from build123d import *

# Parameters (mm, degrees)
SKETCH008_W     = 217
SKETCH008_H     = 40
SKETCH008_W_2   = 214.6
SKETCH008_H_2   = 37.6
PAD006_DEPTH    = 50
SKETCH009_W     = 224.6
SKETCH009_H     = 47.6
SKETCH009_W_2   = 214.6
SKETCH009_H_2   = 37.6
PAD007_DEPTH    = 30
SKETCH010_W     = 224.6
SKETCH010_H     = 20
PAD008_DEPTH    = 5
POCKET001_DEPTH = 87.601
PAD009_DEPTH    = 3
PAD010_DEPTH    = 3


with BuildPart() as part:
    # Sketch008 → Pad006 (new body)
    with BuildSketch(Plane.XY):
        Rectangle(SKETCH008_W, SKETCH008_H)
        Rectangle(SKETCH008_W_2, SKETCH008_H_2, mode=Mode.SUBTRACT)
    extrude(amount=PAD006_DEPTH)

    # Sketch009 → Pad007 (join)
    with BuildSketch(Plane.XY):
        Rectangle(SKETCH009_W, SKETCH009_H)
        Rectangle(SKETCH009_W_2, SKETCH009_H_2, mode=Mode.SUBTRACT)
    extrude(amount=PAD007_DEPTH)

    # Sketch010 → Pad008 (join)
    with BuildSketch(Plane.XY):
        with Locations((0, 33.8)):
            Rectangle(SKETCH010_W, SKETCH010_H)
        with Locations((0, -33.8)):
            Rectangle(SKETCH010_W, SKETCH010_H)
    extrude(amount=PAD008_DEPTH)

    # Sketch011 (on Face1 of Pad008) → Pocket001 (cut, through all)
    with BuildSketch(Plane(origin=(0, 43.8, 0), x_dir=(-1, 0, 0), z_dir=(0, 1, 0))):
        Polygon((-112.3, 30), (-100.3, 0), (-112.3, 0), align=None)
        Polygon((112.3, 30), (89.7, 0), (112.3, 0), align=None)
    extrude(amount=-POCKET001_DEPTH, mode=Mode.SUBTRACT)

    # Sketch012 (on Face5 of Pocket001) → Pad009 (join)
    with BuildSketch(Plane(origin=(-57.224475, 0, -43.109104), x_dir=(0, -1, 0), z_dir=(-0.79872, 0, -0.601703))):
        Polygon((-43.8, 60.232735), (-23.8, 60.232735), (-23.8, 91.532806), (23.8, 91.532806), (23.8, 60.232735), (43.8, 60.232735), (43.8, 53.972721), (-43.8, 53.972721), align=None)
    extrude(amount=-PAD009_DEPTH)

    # Sketch013 (on Face6 of Pad009) → Pad010 (join)
    with BuildSketch(Plane(origin=(86.465517, 0, -34.586207), x_dir=(0, 1, 0), z_dir=(0.928477, 0, -0.371391))):
        Polygon((-23.8, 69.561474), (23.8, 69.561474), (23.8, 42.63565), (43.8, 42.63565), (43.8, 37.250485), (-43.8, 37.250485), (-43.8, 42.63565), (-23.8, 42.63565), align=None)
    extrude(amount=-PAD010_DEPTH)


solid = part.part
Work out the finished part from the listing and answer in its coordinate system (mm). A direction names the side the tool comes from. Round coordinates to 2 decimals unless told otherwise and drop trailing zeros. Order: outer loops, then holes, each group sorted by start corner. A loop starts at its lowest first (then second) coordinate and runs counter-clockwise, first axis right, second up. Notation, with made-up numbers: M 5.25,25 L 17.25,25 A22 ccw 17.25,40 Z; hole C 68.5,0.5 d4. An arc over 180 degrees is marked long. One line per item, written item: value.
Q1. Find section C-C on x = 46.5. Write down the section's boundary in (y, z), then the cut area to 3 significant figures.
Derived:
outline: M -43.8,0 L -18.8,0 L -18.8,50 L -20,50 L -20,30 L -23.8,30 L -23.8,5 L -43.8,5 Z; M 18.8,0 L 43.8,0 L 43.8,5 L 23.8,5 L 23.8,30 L 20,30 L 20,50 L 18.8,50 Z
area: 548 mm²
Q2. Determine the mould class of faces 1 (the face through (106.384, 0.613, 15.21)), 2 (the face through (4, -31, 0)), 3 (the face through (-2, 18.8, 25)) for opening direction X: released by +X, released by -X, zero draft, split by the parting line, or undercut.
Derived:
face 1: released by +X
face 2: zero draft
face 3: undercut
Q3. Find section A-A on y = -16.5. Write down the section's boundary in (x, z).
Derived:
outline: M -112.3,30 L -89.7,0 L -87.3,1.81 L -107.3,28.35 L -107.3,50 L -108.5,50 L -108.5,30 L -108.54,30 L -109.9,31.81 Z; M 97.51,1.11 L 100.3,0 L 112.3,30 L 109.51,31.11 L 109.07,30 L 108.5,30 L 108.5,50 L 107.3,50 L 107.3,25.58 Z
Q4. Straight lines are drawn through the part: line 1 (Y direction, x = -30.5, z = 11); line 2 (Y direction, x = -95.5, z = 40); line 3 (X direction, y = 7, z = 32.5). For each, find the intervals that lie inside material, in ascending order.
Derived:
line 1: -23.8 to -18.8, 18.8 to 23.8
line 2: -20 to -18.8, 18.8 to 20
line 3: -108.5 to -107.3, 107.3 to 108.5
Q5. For faces 4 (the face through (3, 34, 5)), 5 (the face through (4, -43.8, 3)), 6 (the face through (-107.3, 0, 39)), 7 (the face through (-1, 19, 50)), 8 (the face through (3, -34, 5)), determine the directions among +Z, -Z, +X, -X, +Y, -Y from which every point of the face is accessible in a straight line to the end or side of a thin tool.
Derived:
face 4: +Z, +Y
face 5: +Z, -Z, +X, -X, -Y
face 6: +Z
face 7: +Z, +X, -X, +Y, -Y
face 8: +Z, -Y
Q6. Flat-ended cylindrical pins translate along their axes: pin 1 (4 mm diameter, centred on x = -77, z = 23, fed in from -Y); pin 2 (10 mm diameter, centred on x = -31, y = 29, fed in from +Z); pin 3 (8 mm diameter, centred on y = -8.5, z = 12, fed in from +X); pin 4 (3 mm diameter, centred on y = -23, z = 34.5, fed in from +X). Find the tip coordinate at first contact, or state that the pin passes through.
Derived:
pin 1: y = -23.8
pin 2: z = 5
pin 3: x = 106.7
pin 4: through
Q7. Find section B-B on z = 44. Write down the section's boundary in (x, y).
Derived:
outline: M -108.5,-20 L 108.5,-20 L 108.5,20 L -108.5,20 Z; hole M -107.3,-18.8 L 107.3,-18.8 L 107.3,18.8 L -107.3,18.8 Z
